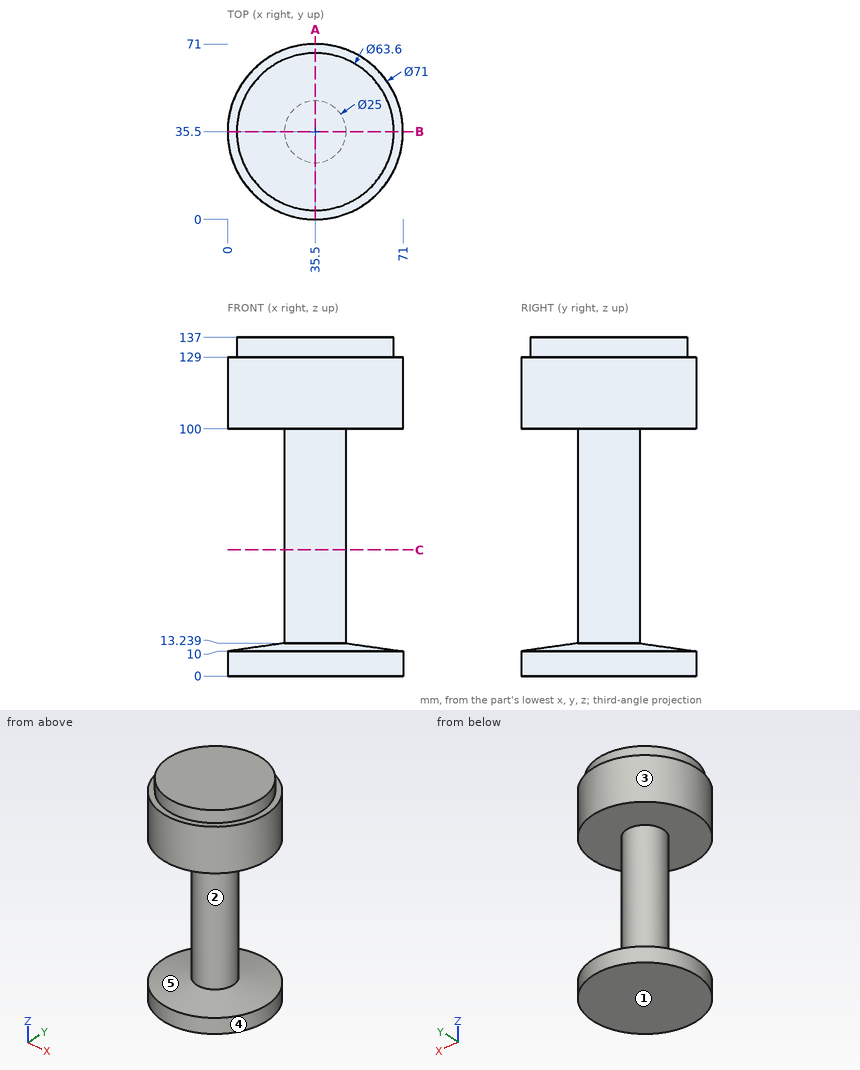
The drawing under review shows one solid part. Ordinate dimensions are in mm from its lowest x, y, z. A direction names the side the tool comes from. Round coordinates to 2 decimals unless told otherwise and drop trailing zeros. Write each loop counter-clockwise with the first axis right and the second up, starting at its lowest first coordinate (ties: lowest second). Pieces come first, ordered by that corner, then holes.
(1) Wall thickness on L1, parallel to Z at x = 57, y = 55; L2, parallel to Z at x = 54, y = 8; L3, parallel to Y at x = 43, z = 94.5: over which ranges is each line inside the solid? List them lowest first.
(2) We need section C-C on z = 51. Give the boundary of the cut face in (x, y).
(3) We need section A-A on x = 35.5. Give the boundary of the cut face in (y, z), and give its area (3 significant figures).
(4) Machinability: for the marked faces 4 and 5, which of the approach directions +Z, -Z, +X, -X, +Y, -Y give a long, thin tool a straight path to every point of the face, cutting with its end or side? Answer none if there is none.
(5) Mouldability with a two-part tool opening along Z and no side actions: class the marked faces 1, 2 and 3 as +Z half, -Z half, draft (parallel to the pull), parting line (faces both ways), or undercut.
(6) Insertion check: pin 1 (4 mm diameter, centred on y = 16, z = 108, fed in from -X); pin 2 (1 mm diameter, centred on x = 41.5, z = 57, fed in from +Y) (1 decimal); pin 3 (8 mm diameter, centred on y = 25.5, z = 111, fed in from -X). Each pin has a flat end and moves straight along its axis. Give the tip position at first contact, or say it passes through.
Findings below:
1. L1: z = 0 to 10.91, 100 to 137
1. L2: z = 0 to 10.33, 100 to 129
1. L3: y = 25.5 to 45.5
2. outline: circle Ø25 at (35.5, 35.5)
3. outline: (0, 0) - (71, 0) - (71, 10) - (48, 13.24) - (48, 100) - (71, 100) - (71, 129) - (67.3, 129) - (67.3, 137) - (3.7, 137) - (3.7, 129) - (0, 129) - (0, 100) - (23, 100) - (23, 13.24) - (0, 10) - close
3. area: 5,600 mm2
4. face 4: +Z, -Z
4. face 5: none
5. face 1: -Z half
5. face 2: undercut
5. face 3: draft
6. pin 1: stops at x = 4.61
6. pin 2: stops at y = 46.7
6. pin 3: stops at x = 0.51
